Geometry: final body of the model. Coordinates: model frame, mm. Coordinates: 2 decimals unless noted, no trailing zeros. Order: outer loops, then holes, each group sorted by start corner. A loop starts at its lowest first (then second) coordinate and runs counter-clockwise, first axis right, second up. Notation, with made-up numbers: M -2.75,-34 L 24.25,-34 A24 ccw 24.25,-21 Z; hole C 41.5,-13.5 d7. An arc over 180 degrees is marked long. Write item = value, one per line. Start each with the question number.
Autodesk Inventor part; units mm, degrees
ref_plane "YZ Plane" through (0, 0, 0) normal (1, 0, 0) x (0, 1, 0)
ref_plane "XZ Plane" through (0, 0, 0) normal (0, 1, 0) x (-1, 0, 0)
ref_plane "XY Plane" through (0, 0, 0) normal (0, 0, 1) x (1, 0, 0)
sketch "Esquisse1" plane through (0, 0, 0) normal (0, 1, 0) x (-1, 0, 0)
  line L0 (57.703, 92.8408) -> (-102.297, 92.8408)
  line L1 (-102.297, -197.1592) -> (57.703, -197.1592)
  line L2 (-102.297, 72.7532) -> (-122.297, 72.7532)
  line L3 (-122.297, 72.7532) -> (-122.297, -177.2468)
  line L4 (-122.297, -177.2468) -> (-102.297, -177.2468)
  line L5 (-102.297, 70.8056) -> (-102.297, 72.7532)
  line L6 (57.703, 70.8056) -> (77.703, 70.8056)
  line L7 (77.703, 70.8056) -> (77.703, -179.1944)
  line L8 (77.703, -179.1944) -> (57.703, -179.1944)
  line L9 (57.703, -179.1944) -> (57.703, -177.2468)
  line L10 (57.703, -197.1592) -> (57.703, -179.1944)
  line L11 (57.703, 70.8056) -> (57.703, 92.8408)
  line L12 (-102.297, 92.8408) -> (-102.297, 72.7532)
  line L13 (-102.297, -177.2468) -> (-102.297, -197.1592)
  point P0 (0, 0)
  dimension "d0" = 290
  dimension "d1" = 160
  dimension "d17" = 20
  dimension "d18" = 250
  dimension "d19" = 20
  dimension "d20" = 250
extrude "Extrusion1" add sketch "Esquisse1" along normal blind 5
ref_plane "Plan de construction1" through (22.297, 0, -197.1592) normal (-1, 0, 0) x (0, 0, 1)
sketch "Sketch2" plane through (0, 5, 0) normal (0, 1, 0) x (1, 0, 0)
  circle A0 centre (60.447, -20.6408) radius 1.5001
  circle A1 centre (60.447, 24.9592) radius 1.5
  circle A2 centre (60.447, 124.9592) radius 1.5
  circle A3 centre (60.447, 79.3592) radius 1.5
  point P0 (0, 0)
extrude "Extrusion2" cut sketch "Sketch2" against normal through all
sketch "Sketch5" plane through (0, 5, 0) normal (0, 1, 0) x (1, 0, 0)
  line L0 (-17.703, -92.8408) -> (62.297, -92.8408)
  line L1 (62.297, -92.8408) -> (62.297, -47.8408)
  line L2 (62.297, -47.8408) -> (-17.703, -47.8408)
  line L3 (-17.703, -47.8408) -> (-17.703, -92.8408)
  line L4 (-57.703, -92.8408) -> (102.297, -92.8408)
  line L5 (-57.703, 197.1592) -> (-57.703, -92.8408)
  line L6 (102.297, -92.8408) -> (102.297, 197.1592)
  line L7 (102.297, 197.1592) -> (-57.703, 197.1592)
  line L8 (-17.703, 197.1592) -> (62.297, 197.1592)
  line L9 (62.297, 197.1592) -> (62.297, 152.1592)
  line L10 (62.297, 152.1592) -> (-17.703, 152.1592)
  line L11 (-17.703, 152.1592) -> (-17.703, 197.1592)
  line L12 (47.297, 152.1592) -> (-17.703, 152.1592)
  line L13 (-17.703, 152.1592) -> (-17.703, 102.1592)
  line L14 (-17.703, 102.1592) -> (47.297, 102.1592)
  line L15 (47.297, 102.1592) -> (47.297, 152.1592)
  point P0 (0, 0)
  dimension "d6" = 0
  dimension "d7" = 45
  dimension "d8" = 40
  dimension "d9" = 40
  dimension "d10" = 40
  dimension "d11" = 40
  dimension "d12" = 45
  dimension "d15" = 65
  dimension "d16" = 50
extrude "Extrusion3" cut sketch "Sketch5" against normal through all contours L3 L2 L1 L0 | L7 L9 L10 L11 | L10 L15 L14 L13
sketch "Sketch6" plane through (0, 5, 0) normal (0, 1, 0) x (1, 0, 0)
  spline S0 degree 3 poles (-57.703, -9.3408) (-57.5164, -9.3408) (-57.3163, -9.3777) (-56.9466, -9.5301) (-56.7768, -9.6456) (-56.51, -9.9124) (-56.3945, -10.0805) (-56.241, -10.4501) (-56.203, -10.6516) (-56.203, -11.03) (-56.241, -11.2314) (-56.3945, -11.601) (-56.51, -11.7692) (-56.7768, -12.0359) (-56.9466, -12.1514) (-57.3163, -12.3038) (-57.5164, -12.3408) (-57.8926, -12.3408) (-58.0946, -12.3027) (-58.4667, -12.1475) (-58.6367, -12.0303) (-58.9007, -11.7625) (-59.0142, -11.5958) (-59.1654, -11.2291) (-59.203, -11.029) (-59.203, -10.6526) (-59.1654, -10.4525) (-59.0142, -10.0858) (-58.9007, -9.9191) (-58.6367, -9.6513) (-58.4667, -9.5341) (-58.0946, -9.3788) (-57.8926, -9.3408) (-57.703, -9.3408) knots 0 0 0 0 0.057709 0.057709 0.115418 0.115418 0.172176 0.172176 0.228935 0.228935 0.285694 0.285694 0.342453 0.342453 0.400161 0.400161 0.45787 0.45787 0.516493 0.516493 0.575116 0.575116 0.631571 0.631571 0.688026 0.688026 0.744481 0.744481 0.800936 0.800936 0.859558 0.859558 0.918181 0.918181 0.918181 0.918181
  spline S1 degree 3 poles (-27.703, -9.3408) (-27.5152, -9.3408) (-27.314, -9.3782) (-26.9424, -9.5324) (-26.772, -9.6492) (-26.5065, -9.9173) (-26.3923, -10.0847) (-26.2405, -10.4525) (-26.203, -10.6528) (-26.203, -11.0288) (-26.2405, -11.229) (-26.3923, -11.5968) (-26.5065, -11.7643) (-26.772, -12.0324) (-26.9424, -12.1492) (-27.314, -12.3034) (-27.5152, -12.3408) (-27.8908, -12.3408) (-28.0911, -12.3034) (-28.4604, -12.1508) (-28.6295, -12.0356) (-28.8953, -11.7698) (-29.0108, -11.6022) (-29.1647, -11.2327) (-29.203, -11.0308) (-29.203, -10.6508) (-29.1647, -10.4489) (-29.0108, -10.0794) (-28.8953, -9.9118) (-28.6295, -9.646) (-28.4604, -9.5307) (-28.0911, -9.3781) (-27.8908, -9.3408) (-27.703, -9.3408) knots 0 0 0 0 0.058071 0.058071 0.116142 0.116142 0.172538 0.172538 0.228935 0.228935 0.285331 0.285331 0.341727 0.341727 0.399798 0.399798 0.457869 0.457869 0.515944 0.515944 0.574019 0.574019 0.631023 0.631023 0.688027 0.688027 0.74503 0.74503 0.802034 0.802034 0.860109 0.860109 0.918184 0.918184 0.918184 0.918184
  point P0 (0, 0)
  point P1 (-57.703, -9.3408)
  point P2 (-27.703, -9.3408)
extrude "Extrusion4" cut sketch "Sketch6" against normal through all
properties part number "etage-bras"
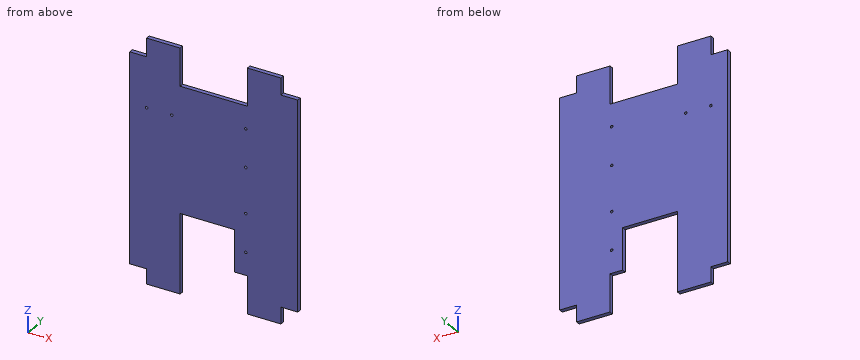
Item 1: Section query A-A on z = -113.5. Output: boundary loops of the cut face in (x, y).
Item 2: First-contact query: pin 1 (2.5 mm diameter, centred on x = 60.45, z = -124.96, fed in from -Y); pin 2 (2.5 mm diameter, centred on y = 3, z = 73, fed in from -X); pin 3 (1.5 mm diameter, centred on x = 53, y = 2.5, fed in from +Z); pin 4 (2.5 mm diameter, centred on x = 11, y = 3, fed in from -Z). Flat tips, straight axial feed; report the tip coordinate or a pass-through.
Item 3: Section query C-C on y = 2.9. Give the number of separate pieces and of enclosed holes in the cut face, and give its area (3 significant figures).
Item 4: Material intervals for probe 1 along X at (y, z) = (4.55, 56); probe 2 along X at (y, z) = (3.15, -136); probe 3 along Z at (x, y) = (2.5, 2.75), sorted ascending. Write a range as [from, to].
Item 5: Section query B-B on x = 1. Output: boundary loops of the cut face in (y, z), and give its area (3 significant figures).
Ans:
q1.outline = M -77.7,0 L -17.7,0 L -17.7,5 L -77.7,5 Z; M 47.3,0 L 122.3,0 L 122.3,5 L 47.3,5 Z
q2.pin_1 = through
q2.pin_2 = -57.7
q2.pin_3 = 47.84
q2.pin_4 = -102.16
q3.separate_pieces = 1
q3.enclosed_holes = 6
q3.area = 45,900 mm^2
q4.probe_1 = [-77.7, -17.7], [62.3, 122.3]
q4.probe_2 = [-77.7, -17.7], [47.3, 122.3]
q4.probe_3 = [-102.16, 47.84]
q5.outline = M 0,-102.16 L 5,-102.16 L 5,47.84 L 0,47.84 Z
q5.area = 750 mm^2
